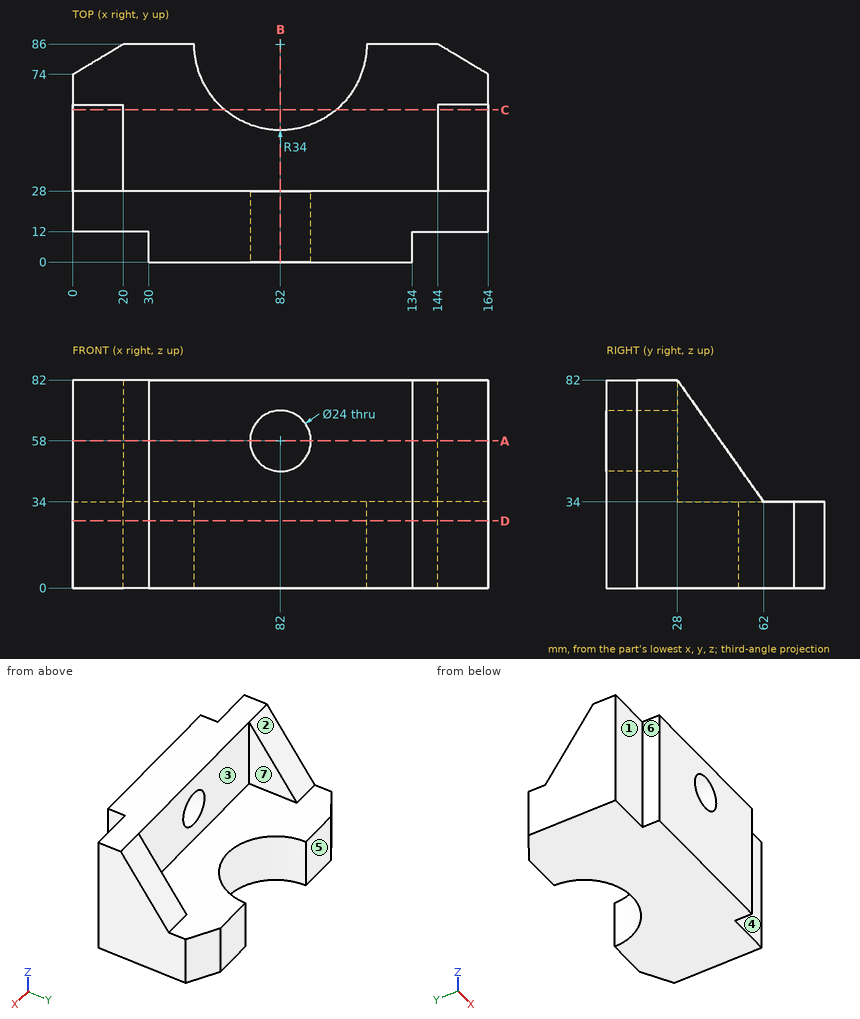
Design review of the part shown in the three views and the two pictorial views. Dimensions are in mm from the part's minimum x, y and z. A direction names the side the tool comes from. Coordinates: 2 decimals unless noted, no trailing zeros. Loops run counter-clockwise (first coordinate to the right, second up) from the corner with the lowest first, then second, coordinate; pieces in that order, holes last.
Q1. The part is to be moulded in two halves that separate along X. For the marked faces 5, 6 and 7, say which applies: +X half, -X half, draft (parallel to the pull), parting line (faces both ways), or undercut.
Reported:
face 5: draft
face 6: -X half
face 7: undercut
Q2. To check wall thickness, follow line 1 (Z direction, x = 82, y = 12.5); line 2 (X direction, y = 52.5, z = 36); line 3 (Y direction, x = 38, z = 54.5). State the ranges of each line that lie inside material, in increasing order.
Reported:
line 1: z = 0 to 46, 70 to 82
line 2: x = 0 to 20, 144 to 164
line 3: y = 0 to 28
Q3. We need section C-C on y = 60. State the section outline as (x, z) points, and give its area (3 significant figures).
Reported:
outline: (0, 0) - (60.09, 0) - (60.09, 34) - (20, 34) - (20, 36.82) - (0, 36.82) - close; (103.91, 0) - (164, 0) - (164, 36.82) - (144, 36.82) - (144, 34) - (103.91, 34) - close
area: 4,200 mm2
Q4. For pin 1 (10 mm diameter, centred on x = 30.5, z = 73, fed in from +Y); pin 2 (12 mm diameter, centred on y = 29.5, z = 39, fed in from -X); pin 3 (13 mm diameter, centred on y = 4.5, z = 30, fed in from -X); pin 4 (8 mm diameter, centred on x = 47.5, y = 56, fed in from +Z), all flat-tipped, find the tip position at first contact; note any pin that passes through.
Reported:
pin 1: stops at y = 28
pin 2: stops at x = 0
pin 3: stops at x = 30
pin 4: stops at z = 34
Q5. We need section D-D on z = 26.5. State the section outline as (x, y) points, and give its area (3 significant figures).
Reported:
outline: (0, 12) - (30, 12) - (30, 0) - (134, 0) - (134, 12) - (164, 12) - (164, 74) - (144, 86) - (116, 86) arc R34 cw to (48, 86) - (20, 86) - (0, 74) - close
area: 11,300 mm2
Q6. We need section B-B on x = 82. State the section outline as (y, z) points, and give its area (3 significant figures).
Reported:
outline: (0, 0) - (52, 0) - (52, 34) - (28, 34) - (28, 46) - (0, 46) - close; (0, 70) - (28, 70) - (28, 82) - (0, 82) - close
area: 2,440 mm2
Q7. Tool access review of the marked faces 1, 2, 3 and 4: name each direction out of +Z, -Z, +X, -X, +Y, -Y from which nothing blocks a thin tool from reaching the whole face with its end or side.
Reported:
face 1: +Z, -Z, -X, -Y
face 2: +Z, +X, -X, +Y
face 3: +Z, +Y
face 4: +Z, -Z, +X, -Y
Q8. We need section A-A on z = 58. State the section outline as (x, y) points, and give its area (3 significant figures).
Reported:
outline: (0, 12) - (30, 12) - (30, 0) - (70, 0) - (70, 28) - (20, 28) - (20, 45) - (0, 45) - close; (94, 0) - (134, 0) - (134, 12) - (164, 12) - (164, 45) - (144, 45) - (144, 28) - (94, 28) - close
area: 3,880 mm2
